Autodesk Inventor part; units mm, degrees
ref_plane "YZ Plane" through (0, 0, 0) normal (1, 0, 0) x (0, 1, 0)
ref_plane "XZ Plane" through (0, 0, 0) normal (0, 1, 0) x (-1, 0, 0)
ref_plane "XY Plane" through (0, 0, 0) normal (0, 0, 1) x (1, 0, 0)
sketch "Sketch1" plane through (0, 0, 0) normal (0, 0, 1) x (1, 0, 0)
  line L0 (0, 0) -> (23, 0)
  line L1 (23, 0) -> (23, -14.8)
  line L2 (23, -14.8) -> (0, -14.8)
  line L3 (0, -14.8) -> (0, 0)
  circle A0 centre (5.65, -4.5) radius 1.5
  circle A1 centre (17.35, -4.5) radius 1.5
  circle A2 centre (11.5, -9.8) radius 2.5
  dimension "d0" = 23
  dimension "d1" = 14.8
  dimension "d2" = 4.5
  dimension "d3" = 11.7
  dimension "d4" = 5.65
  dimension "d5" = 5.65
  dimension "d6" = 11.5
  dimension "d7" = 5
  dimension "d8" = 3
  dimension "d9" = 3
  dimension "d10" = 5
extrude "Extrusion1" add sketch "Sketch1" along normal blind 6
sketch "Sketch2" plane through (0, 0, 0) normal (0, 0, -1) x (-1, 0, 0)
  circle A0 centre (-17.35, -4.5) radius 1.5
  circle A1 centre (-17.35, -4.5) radius 2.5
  circle A2 centre (-5.65, -4.5) radius 1.5
  circle A3 centre (-5.65, -4.5) radius 2.5
  point P0 (0, 0)
  dimension "d13" = 5
  dimension "d14" = 5
extrude "Extrusion2" cut sketch "Sketch2" against normal blind 4
equation "\"d9\" = d8"
equation "\"d14\" = d13"
properties part number "cam m6 replacement v01"
For this review, take the finished solid that the model builds, in its own axes (mm). A direction names the side the tool comes from. Give positions to 0.01 mm unless a question says otherwise; leave off trailing zeros. Order: outer loops, then holes, each group sorted by start corner. A loop starts at its lowest first (then second) coordinate and runs counter-clockwise, first axis right, second up. Notation, with made-up numbers: (70.5, -25) - (83.5, -25) arc R14 ccw to (83.5, -12) - close; hole circle Ø5 at (27.5, 33.5). An arc over 180 degrees is marked (long way). Answer as a JSON object with one key per item and string values. Group by question number.
Item 1: Draft analysis for pull direction Y (two halves, no side actions). For faces 1 (the flat face through (11, -7, 6)), 2 (the flat face through (12, -14.8, 3)), 3 (the cylindrical face through (6.456, -5.765, 4.986)), state which applies: pulls with the +Y half, pulls with the -Y half, needs draft (parallel to the pull), parting line crosses it, or undercut.
Item 2: Wall thickness on line 1 along X through (y, z) = (-4.5, 4.7); line 2 along Y through (x, z) = (5.65, 1.8); line 3 along X through (y, z) = (-5.75, 1.4): over which ranges is each line inside the solid? List them lowest first.
Item 3: Clearance check with flat-ended pins moving along their axes: pin 1 Ø6.5 at (x, y) = (5.65, -4.5) entering from +Z; pin 2 Ø1.5 at (x, y) = (5, -3.5) entering from -Z; pin 3 Ø1.5 at (x, y) = (17.5, -4) entering from -Z. State where each tip first meets the part, or that it passes through.
Item 4: Machinability: for faces 4 (the cylindrical face through (14.965, -3.749, 1.972)), 5 (the flat face through (11, 0, 3)), which of the approach directions +Z, -Z, +X, -X, +Y, -Y give a long, thin tool a straight path to every point of the face, cutting with its end or side? Answer none if there is none.
Item 5: Take a section at B-B on z = 4.65. Give the boundary of the cut face in (x, y), and give its area (3 significant figures).
Item 6: Take a section at D-D on y = -9.8. Give the boundary of the cut face in (x, z), and give its area (3 significant figures).
Item 7: Take a section at A-A on y = -4.5. Give the boundary of the cut face in (x, z), and give its area (3 significant figures).
Item 8: Take a section at C-C on x = 17.25. Give the boundary of the cut face in (y, z), and give its area (3 significant figures).
Reported:
{
 "1": {"face 1": "needs draft", "face 2": "pulls with the -Y half", "face 3": "undercut"},
 "2": {"line 1": "0 to 4.15, 7.15 to 15.85, 18.85 to 23", "line 2": "-14.8 to -7, -2 to 0", "line 3": "0 to 3.48, 7.82 to 15.18, 19.52 to 23"},
 "3": {"pin 1": "z = 6", "pin 2": "z = 4", "pin 3": "through"},
 "4": {"face 4": "-Z", "face 5": "+Z, -Z, +X, -X, +Y"},
 "5": {"outline": "(0, -14.8) - (23, -14.8) - (23, 0) - (0, 0) - close; hole circle Ø3 at (5.65, -4.5); hole circle Ø5 at (11.5, -9.8); hole circle Ø3 at (17.35, -4.5)", "area": "307 mm^2"},
 "6": {"outline": "(0, 0) - (9, 0) - (9, 6) - (0, 6) - close; (14, 0) - (23, 0) - (23, 6) - (14, 6) - close", "area": "108 mm^2"},
 "7": {"outline": "(0, 0) - (3.15, 0) - (3.15, 4) - (4.15, 4) - (4.15, 6) - (0, 6) - close; (7.15, 4) - (8.15, 4) - (8.15, 0) - (14.85, 0) - (14.85, 4) - (15.85, 4) - (15.85, 6) - (7.15, 6) - close; (18.85, 4) - (19.85, 4) - (19.85, 0) - (23, 0) - (23, 6) - (18.85, 6) - close", "area": "86.0 mm^2"},
 "8": {"outline": "(-14.8, 0) - (-7, 0) - (-7, 4) - (-6, 4) - (-6, 6) - (-14.8, 6) - close; (-3, 4) - (-2, 4) - (-2, 0) - (0, 0) - (0, 6) - (-3, 6) - close", "area": "62.8 mm^2"}
}
